Verification items for the finished model (mm, model axes). A direction names the side the tool comes from. Round coordinates to 2 decimals unless told otherwise and drop trailing zeros. Order: outer loops, then holes, each group sorted by start corner. A loop starts at its lowest first (then second) coordinate and runs counter-clockwise, first axis right, second up. Notation, with made-up numbers: (-37.5, 81.25) -> (20.5, 81.25) arc R23 ccw to (20.5, 115.25) -> close; hole circle Ø11 at (-16, 54). An arc over 180 degrees is marked (long way). Return JSON: item names as keys, results as strings. Group by question number.
1) Scan lines: L1, parallel to Z at x = -34, y = 66; L2, parallel to Y at x = -2, z = 8.25; L3, parallel to Y at x = -17, z = 4.5. Record each from-to range of solid material in increasing order.
2) Section check C-C on x = -2. Enter the section's corners in (y, z), plus the area to 3 significant figures.
3) Section check D-D on y = 63. Enter the section's corners in (x, z).
4) Tool access check on faces 5 (the cylindrical face through (-3.04, 46.75, 7.04)), 6 (the flat face through (-18, 59, 11)), 7 (the flat face through (-17.9, 58.7, 2.6)), 8 (the flat face through (-15, 34, 2)). Record the directions out of +Z, -Z, +X, -X, +Y, -Y that give a thin tool (end or side, any length) a straight path to the whole face; none if there is none.
5) Section check B-B on x = -12. Enter the section's corners in (y, z), plus the area to 3 significant figures.
6) Draft check along Y on faces 1 (the flat face through (-3, 8, 5.25)), 2 (the flat face through (-3, 42, 8.75)), 3 (the cylindrical face through (-6.6, 50.43, 6.93)), 4 (the flat face through (-18, 59, 1)). Enter one of: pulls with the +Y half, pulls with the -Y half, needs draft (parallel to the pull), parting line crosses it, or undercut.
7) Section check A-A on y = 39. Enter the section's corners in (x, z), plus the area to 3 significant figures.
8) Depth check by flat-ended pin: pin 1 (0.7 mm diameter, centred on x = -20.5, z = 1.5, fed in from +Y); pin 2 (3 mm diameter, centred on y = 56.5, z = 7, fed in from +X); pin 3 (5.5 mm diameter, centred on x = -2, y = 8.5, fed in from -Z); pin 4 (2 mm diameter, centred on y = 20.5, z = 7.5, fed in from -X). Enter the tip coordinate at first touch or a pass-through.
```python
from build123d import *

# Parameters (mm, degrees)
F1_DEPTH = 12
F2_DEPTH = 2
F5_DEPTH = 6
F6_R     = 1.75
F7_DEPTH = 6
F9_DEPTH = 30.001


with BuildPart() as f1:
    # F0 (on Top) → F1 (new body)
    with BuildSketch(Plane.XY):
        with BuildLine():
            Line((-6, 0), (0, 0))
            Line((0, 0), (0, 51))
            ThreePointArc((0, 51), (-2.343146, 56.656854), (-8, 59))
            Line((-8, 59), (-28, 59))
            ThreePointArc((-28, 59), (-29.414214, 59.585786), (-30, 61))
            Line((-30, 61), (-30, 72))
            Line((-30, 72), (-36, 72))
            Line((-36, 72), (-36, 59))
            ThreePointArc((-36, 59), (-35.766593, 57.081659), (-35.079992, 55.275257))
            ThreePointArc((-35.079992, 55.275257), (-32.135339, 52.151718), (-28, 51))
            Line((-28, 51), (-8, 51))
            ThreePointArc((-8, 51), (-6.585786, 50.414214), (-6, 49))
            Line((-6, 49), (-6, 0))
        make_face()
    extrude(amount=F1_DEPTH)

    # F0 (on Top) → F2 (join)
    with BuildSketch(Plane.XY):
        with BuildLine():
            Line((-35.079992, 55.275257), (-6, 0))
            Line((-6, 0), (-6, 49))
            ThreePointArc((-6, 49), (-6.585786, 50.414214), (-8, 51))
            Line((-8, 51), (-28, 51))
            ThreePointArc((-28, 51), (-32.135339, 52.151718), (-35.079992, 55.275257))
        make_face()
    extrude(amount=F2_DEPTH)

    # F4 (on face) → F5 (cut, through all)
    with BuildSketch(Plane(origin=(-6, 0, 0), x_dir=(0, -1, 0), z_dir=(-1, 0, 0))):
        with BuildLine():
            ThreePointArc((-5, 12), (-1.464466, 10.535534), (0, 7))
            Line((0, 7), (0, 12))
            Line((0, 12), (-5, 12))
        make_face()
        with BuildLine():
            ThreePointArc((-5, 5.25), (-3.25, 7), (-5, 8.75))
            Line((-5, 8.75), (-10, 8.75))
            ThreePointArc((-10, 8.75), (-11.75, 7), (-10, 5.25))
            Line((-10, 5.25), (-5, 5.25))
        make_face()
        with BuildLine():
            ThreePointArc((-40, 5.25), (-38.25, 7), (-40, 8.75))
            Line((-40, 8.75), (-45, 8.75))
            ThreePointArc((-45, 8.75), (-46.75, 7), (-45, 5.25))
            Line((-45, 5.25), (-40, 5.25))
        make_face()
    extrude(amount=-F5_DEPTH, mode=Mode.SUBTRACT)

    # F6 (on face) → F7 (cut, through all)
    with BuildSketch(Plane(origin=(-36, 0, 0), x_dir=(0, -1, 0), z_dir=(-1, 0, 0))):
        with Locations((-66, 6)):
            Circle(F6_R)
        with BuildLine():
            ThreePointArc((-72, 6), (-70.242641, 10.242641), (-66, 12))
            Line((-66, 12), (-72, 12))
            Line((-72, 12), (-72, 6))
        make_face()
        with BuildLine():
            ThreePointArc((-66, 0), (-70.242641, 1.757359), (-72, 6))
            Line((-72, 6), (-72, 0))
            Line((-72, 0), (-66, 0))
        make_face()
    extrude(amount=-F7_DEPTH, mode=Mode.SUBTRACT)

    # F8 (on face) → F9 (cut, through all)
    with BuildSketch(Plane.YZ.offset(-30)):
        Polygon((66, 16.7), (57.8, 8.5), (57.8, 3.5), (66, -4.7), align=None)
    extrude(amount=F9_DEPTH, mode=Mode.SUBTRACT)


solid = f1.part
```
Check result:
{
 "1": {"L1": "0 to 4.25, 7.75 to 12", "L2": "0.16 to 3.78, 11.22 to 38.78, 46.22 to 56.29", "L3": "51 to 57.8"},
 "2": {"outline": "(0, 0) -> (56.29, 0) -> (56.29, 12) -> (5, 12) arc R5 ccw to (0, 7) -> close; hole (5, 5.25) -> (10, 5.25) arc R1.75 ccw to (10, 8.75) -> (5, 8.75) arc R1.75 ccw to start; hole (40, 5.25) -> (45, 5.25) arc R1.75 ccw to (45, 8.75) -> (40, 8.75) arc R1.75 ccw to start", "area": "616 mm^2"},
 "3": {"outline": "(-36, 0) -> (-30, 0) -> (-30, 12) -> (-36, 12) -> close"},
 "4": {"face 5": "+X, -X", "face 6": "+Z, -Z, +X, +Y", "face 7": "+X, +Y", "face 8": "+Z, -X, -Y"},
 "5": {"outline": "(11.4, 0) -> (59, 0) -> (59, 2.3) -> (57.8, 3.5) -> (57.8, 8.5) -> (59, 9.7) -> (59, 12) -> (51, 12) -> (51, 2) -> (11.4, 2) -> close", "area": "168 mm^2"},
 "6": {"face 1": "undercut", "face 2": "undercut", "face 3": "pulls with the -Y half", "face 4": "pulls with the +Y half"},
 "7": {"outline": "(-26.52, 0) -> (0, 0) -> (0, 5.56) -> (-6, 5.56) -> (-6, 2) -> (-26.52, 2) -> close; (-6, 8.44) -> (0, 8.44) -> (0, 12) -> (-6, 12) -> close", "area": "95.8 mm^2"},
 "8": {"pin 1": "y = 59", "pin 2": "x = -1.07", "pin 3": "z = 0", "pin 4": "x = -6"}
}
